Input: part model. Units: mm. Frame: model coordinates. Face numbers are marked on the shaded views. Round coordinates to 2 decimals unless told otherwise and drop trailing zeros. Loops run counter-clockwise (first coordinate to the right, second up) from the corner with the lowest first, then second, coordinate; pieces in that order, holes last. Notation, with made-up numbers: M -15.5,65 L 43.5,65 A19 cw 43.5,70 Z; hole C 53.25,47 d1. An arc over 180 degrees is marked long. Put each result on its own line as item: value. Start each with the question number.
1) Draft query along Y for the marked faces 1 and 2. Return one class per face: +Y half, -Y half, draft (parallel to the pull), parting line (faces both ways), or undercut.
2) Section A-A on x = 18.5. Output: boundary loops of the cut face in (y, z), plus the area to 3 significant figures.
3) Section B-B on y = 25. Output: boundary loops of the cut face in (x, z), plus the area to 3 significant figures.
4) Pin query (flat end, axial travel): pin 1 (0.5 mm diameter, centred on x = 40.5, z = 0, fed in from -Y); pin 2 (0.5 mm diameter, centred on x = 40.5, z = 0, fed in from +Y); pin 3 (1.1 mm diameter, centred on y = 18, z = -0.5, fed in from -X); pin 4 (1.3 mm diameter, centred on x = -11.34, y = 45.37, fed in from -Z). Return the tip coordinate at first contact, or that it passes through.
5) Line query: probe 1 along X at (y, z) = (-3.5, -0.55); probe 2 along Y at (x, z) = (31.5, -0.5); probe 3 along Z at (x, y) = (22, -1.5). Output: solid intervals per line, ascending.
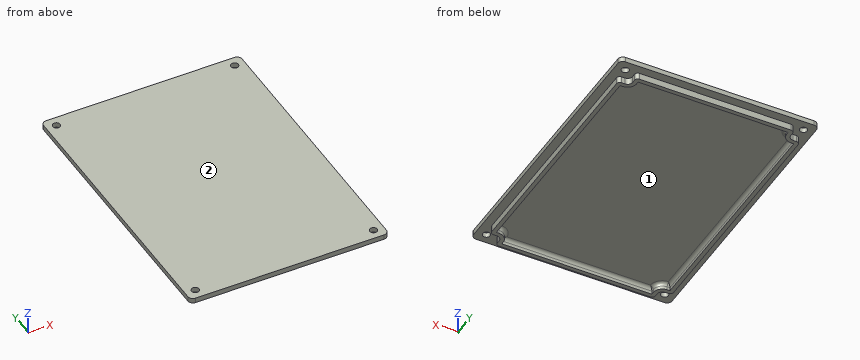
from build123d import *

# Parameters (mm, degrees)
LID_BASE_DEPTH = 1.5
INSERT_DEPTH   = 2
CONG_1_R       = 1
M3_HOLE_REACH  = 67.94
ESQUISSE5_R    = 1.1


with BuildPart() as part:
    # Esquisse3 → Lid_Base (new body)
    with BuildSketch(Plane.XY.offset(1)):
        with BuildLine():
            Line((-14.335501752, 46.874395923), (-14.335501752, -33.705604077))
            ThreePointArc((-14.335501752, -33.705604077), (-13.896161923, -34.766264249), (-12.835501752, -35.205604077))
            Line((-12.835501752, -35.205604077), (43.174498248, -35.205604077))
            ThreePointArc((43.174498248, -35.205604077), (44.23515842, -34.766264249), (44.674498248, -33.705604077))
            Line((44.674498248, -33.705604077), (44.674498248, 46.874395923))
            ThreePointArc((44.674498248, 46.874395923), (44.23515842, 47.935056095), (43.174498248, 48.374395923))
            Line((43.174498248, 48.374395923), (-12.835501752, 48.374395923))
            ThreePointArc((-12.835501752, 48.374395923), (-13.896161923, 47.935056095), (-14.335501752, 46.874395923))
        make_face()
    extrude(amount=LID_BASE_DEPTH)

    # Esquisse4 → Insert (add)
    with BuildSketch(Plane(origin=(0, 0, 1), x_dir=(-1, 0, 0), z_dir=(0, 0, -1))):
        with BuildLine():
            Line((7.335501752, 45.874395923), (-37.674498248, 45.874395923))
            ThreePointArc((-37.674498248, 45.874395923), (-38.38160503, 45.581502704), (-38.674498248, 44.874395923))
            Line((-38.674498248, 44.874395923), (-38.674498248, 43.874395923))
            ThreePointArc((-38.674498248, 43.874395923), (-39.113838077, 42.813735751), (-40.174498248, 42.374395923))
            Line((-40.174498248, 42.374395923), (-41.174498248, 42.374395923))
            ThreePointArc((-41.174498248, 42.374395923), (-41.88160503, 42.081502704), (-42.174498248, 41.374395923))
            Line((-42.174498248, 41.374395923), (-42.174498248, -28.205604077))
            ThreePointArc((-42.174498248, -28.205604077), (-41.88160503, -28.912710858), (-41.174498248, -29.205604077))
            Line((-41.174498248, -29.205604077), (-40.174498248, -29.205604077))
            ThreePointArc((-40.174498248, -29.205604077), (-39.113838077, -29.644943905), (-38.674498248, -30.705604077))
            Line((-38.674498248, -30.705604077), (-38.674498248, -31.705604077))
            ThreePointArc((-38.674498248, -31.705604077), (-38.38160503, -32.412710858), (-37.674498248, -32.705604077))
            Line((-37.674498248, -32.705604077), (7.335501752, -32.705604077))
            ThreePointArc((7.335501752, -32.705604077), (8.042608533, -32.412710858), (8.335501752, -31.705604077))
            Line((8.335501752, -31.705604077), (8.335501752, -30.705604077))
            ThreePointArc((8.335501752, -30.705604077), (8.77484158, -29.644943905), (9.835501752, -29.205604077))
            Line((9.835501752, -29.205604077), (10.835501752, -29.205604077))
            ThreePointArc((10.835501752, -29.205604077), (11.542608533, -28.912710858), (11.835501752, -28.205604077))
            Line((11.835501752, -28.205604077), (11.835501752, 41.374395923))
            ThreePointArc((11.835501752, 41.374395923), (11.542608533, 42.081502704), (10.835501752, 42.374395923))
            Line((10.835501752, 42.374395923), (9.835501752, 42.374395923))
            ThreePointArc((9.835501752, 42.374395923), (8.77484158, 42.813735751), (8.335501752, 43.874395923))
            Line((8.335501752, 43.874395923), (8.335501752, 44.874395923))
            ThreePointArc((8.335501752, 44.874395923), (8.042608533, 45.581502704), (7.335501752, 45.874395923))
        make_face()
        with BuildLine():
            Line((7.135501752, 44.674395923), (-37.474498248, 44.674395923))
            Line((-37.474498248, 44.674395923), (-37.474498248, 43.874395923))
            ThreePointArc((-37.474498248, 43.874395923), (-38.265309939, 41.965207614), (-40.174498248, 41.174395923))
            Line((-40.174498248, 41.174395923), (-40.974498248, 41.174395923))
            Line((-40.974498248, 41.174395923), (-40.974498248, -28.005604077))
            Line((-40.974498248, -28.005604077), (-40.174498248, -28.005604077))
            ThreePointArc((-40.174498248, -28.005604077), (-38.265309939, -28.796415768), (-37.474498248, -30.705604077))
            Line((-37.474498248, -30.705604077), (-37.474498248, -31.505604077))
            Line((-37.474498248, -31.505604077), (7.135501752, -31.505604077))
            Line((7.135501752, -31.505604077), (7.135501752, -30.705604077))
            ThreePointArc((7.135501752, -30.705604077), (7.926313442, -28.796415768), (9.835501752, -28.005604077))
            Line((9.835501752, -28.005604077), (10.635501752, -28.005604077))
            Line((10.635501752, -28.005604077), (10.635501752, 41.174395923))
            Line((10.635501752, 41.174395923), (9.835501752, 41.174395923))
            ThreePointArc((9.835501752, 41.174395923), (7.926313442, 41.965207614), (7.135501752, 43.874395923))
            Line((7.135501752, 43.874395923), (7.135501752, 44.674395923))
        make_face(mode=Mode.SUBTRACT)
    extrude(amount=INSERT_DEPTH)

    # Congé1
    # the kernel refuses this fillet: 1 mm, written as the material it adds along each edge
    with BuildSketch(Plane(origin=(-10.635501752, -28.005604077, 1), x_dir=(0, 0, -1), z_dir=(0, 1, 0)), Plane(origin=(40.974498248, 41.174395923, 1), x_dir=(0, 0, -1), z_dir=(0, -1, 0))) as cong_1_piece_1:
        with BuildLine():
            CenterArc((CONG_1_R, -CONG_1_R), CONG_1_R, 90, 90)
            Line((0, -CONG_1_R), (0, 0))
            Line((0, 0), (CONG_1_R, 0))
        make_face()
    extrude(amount=69.18)
    with BuildSketch(Plane(origin=(-9.835501752, -30.705604077, 1), x_dir=(1, 0, 0), z_dir=(0, -1, 0))) as cong_1_piece_2:
        with BuildLine():
            CenterArc((2.7 + CONG_1_R, -CONG_1_R), CONG_1_R, 90, 90)
            Line((2.7 + CONG_1_R, 0), (2.7, 0))
            Line((2.7, 0), (2.7, -CONG_1_R))
        make_face()
    revolve(axis=Axis((-9.835501752, -30.705604077, 1), (0, 0, 1)), revolution_arc=90)
    with BuildSketch(Plane(origin=(37.474498248, -31.505604077, 1), x_dir=(0, 0, -1), z_dir=(-1, 0, 0)), Plane(origin=(-7.135501752, 44.674395923, 1), x_dir=(0, 0, -1), z_dir=(1, 0, 0))) as cong_1_piece_3:
        with BuildLine():
            CenterArc((CONG_1_R, -CONG_1_R), CONG_1_R, 90, 90)
            Line((0, -CONG_1_R), (0, 0))
            Line((0, 0), (CONG_1_R, 0))
        make_face()
    extrude(amount=44.61)
    with BuildSketch(Plane(origin=(40.174498248, -30.705604077, 1), x_dir=(0, 1, 0), z_dir=(1, 0, 0))) as cong_1_piece_4:
        with BuildLine():
            CenterArc((2.7 + CONG_1_R, -CONG_1_R), CONG_1_R, 90, 90)
            Line((2.7 + CONG_1_R, 0), (2.7, 0))
            Line((2.7, 0), (2.7, -CONG_1_R))
        make_face()
    revolve(axis=Axis((40.174498248, -30.705604077, 1), (0, 0, 1)), revolution_arc=90)
    with BuildSketch(Plane(origin=(40.174498248, 43.874395923, 1), x_dir=(-1, 0, 0), z_dir=(0, 1, 0))) as cong_1_piece_5:
        with BuildLine():
            CenterArc((2.7 + CONG_1_R, -CONG_1_R), CONG_1_R, 90, 90)
            Line((2.7 + CONG_1_R, 0), (2.7, 0))
            Line((2.7, 0), (2.7, -CONG_1_R))
        make_face()
    revolve(axis=Axis((40.174498248, 43.874395923, 1), (0, 0, 1)), revolution_arc=90)
    with BuildSketch(Plane(origin=(-9.835501752, 43.874395923, 1), x_dir=(0, -1, 0), z_dir=(-1, 0, 0))) as cong_1_piece_6:
        with BuildLine():
            CenterArc((2.7 + CONG_1_R, -CONG_1_R), CONG_1_R, 90, 90)
            Line((2.7 + CONG_1_R, 0), (2.7, 0))
            Line((2.7, 0), (2.7, -CONG_1_R))
        make_face()
    revolve(axis=Axis((-9.835501752, 43.874395923, 1), (0, 0, 1)), revolution_arc=90)
    with BuildSketch(Plane(origin=(-10.635501752, 41.174395923, 1), x_dir=(0, 0, -1), z_dir=(1, 0, 0)), Plane(origin=(-7.135501752, 43.874395923, 1), x_dir=(0, 0, -1), z_dir=(0, 1, 0)), Plane(origin=(37.474498248, 44.674395923, 1), x_dir=(0, 0, -1), z_dir=(0, -1, 0)), Plane(origin=(40.174498248, 41.174395923, 1), x_dir=(0, 0, -1), z_dir=(1, 0, 0)), Plane(origin=(40.974498248, -28.005604077, 1), x_dir=(0, 0, -1), z_dir=(-1, 0, 0)), Plane(origin=(37.474498248, -30.705604077, 1), x_dir=(0, 0, -1), z_dir=(0, -1, 0)), Plane(origin=(-7.135501752, -31.505604077, 1), x_dir=(0, 0, -1), z_dir=(0, 1, 0)), Plane(origin=(-9.835501752, -28.005604077, 1), x_dir=(0, 0, -1), z_dir=(-1, 0, 0))) as cong_1_piece_7:
        with BuildLine():
            CenterArc((CONG_1_R, -CONG_1_R), CONG_1_R, 90, 90)
            Line((0, -CONG_1_R), (0, 0))
            Line((0, 0), (CONG_1_R, 0))
        make_face()
    extrude(amount=0.8)

    # Esquisse5 → M3_Hole (cut, up to next)
    with BuildSketch(Plane.XY.offset(2.5), mode=Mode.PRIVATE) as m3_hole_sk1:
        with Locations((-11.335501752, -32.205604077)):
            Circle(ESQUISSE5_R)
    m3_hole_tool1 = extrude(m3_hole_sk1.sketch, amount=-M3_HOLE_REACH, mode=Mode.PRIVATE) & part.part
    # Esquisse5 → M3_Hole (cut, up to next)
    with BuildSketch(Plane.XY.offset(2.5), mode=Mode.PRIVATE) as m3_hole_sk2:
        with Locations((-11.335501752, 45.374395923)):
            Circle(ESQUISSE5_R)
    m3_hole_tool2 = extrude(m3_hole_sk2.sketch, amount=-M3_HOLE_REACH, mode=Mode.PRIVATE) & part.part
    # Esquisse5 → M3_Hole (cut, up to next)
    with BuildSketch(Plane.XY.offset(2.5), mode=Mode.PRIVATE) as m3_hole_sk3:
        with Locations((41.674498248, 45.374395923)):
            Circle(ESQUISSE5_R)
    m3_hole_tool3 = extrude(m3_hole_sk3.sketch, amount=-M3_HOLE_REACH, mode=Mode.PRIVATE) & part.part
    # Esquisse5 → M3_Hole (cut, up to next)
    with BuildSketch(Plane.XY.offset(2.5), mode=Mode.PRIVATE) as m3_hole_sk4:
        with Locations((41.674498248, -32.205604077)):
            Circle(ESQUISSE5_R)
    m3_hole_tool4 = extrude(m3_hole_sk4.sketch, amount=-M3_HOLE_REACH, mode=Mode.PRIVATE) & part.part
    add(m3_hole_tool1.solids().sort_by_distance((-11.335502, -32.205604, 2.5))[0], mode=Mode.SUBTRACT)
    add(m3_hole_tool2.solids().sort_by_distance((-11.335502, 45.374396, 2.5))[0], mode=Mode.SUBTRACT)
    add(m3_hole_tool3.solids().sort_by_distance((41.674498, 45.374396, 2.5))[0], mode=Mode.SUBTRACT)
    add(m3_hole_tool4.solids().sort_by_distance((41.674498, -32.205604, 2.5))[0], mode=Mode.SUBTRACT)


solid = part.part
Geometry results:
1. face 1: undercut
1. face 2: draft
2. outline: M -35.21,1 L -32.71,1 L -32.71,-1 L -31.51,-1 L -31.51,0 A1 cw -30.51,1 L 43.67,1 A1 cw 44.67,0 L 44.67,-1 L 45.87,-1 L 45.87,1 L 48.37,1 L 48.37,2.5 L -35.21,2.5 Z
2. area: 131 mm²
3. outline: M -14.34,1 L -11.84,1 L -11.84,-1 L -10.64,-1 L -10.64,0 A1 cw -9.64,1 L 39.97,1 A1 cw 40.97,0 L 40.97,-1 L 42.17,-1 L 42.17,1 L 44.67,1 L 44.67,2.5 L -14.34,2.5 Z
3. area: 93.7 mm²
4. pin 1: stops at y = -29.21
4. pin 2: stops at y = 42.37
4. pin 3: stops at x = -11.84
4. pin 4: passes through
5. probe 1: x = -11.84 to -10.64, 40.97 to 42.17
5. probe 2: y = -32.71 to -31.51, 44.67 to 45.87
5. probe 3: z = 1 to 2.5
